Here's the drawing with two shaded views (mm, measured from the low corner). I have some questions. A direction names the side the tool comes from. Round coordinates to 2 decimals unless told otherwise and drop trailing zeros. Write each loop counter-clockwise with the first axis right and the second up, starting at its lowest first coordinate (ties: lowest second). Pieces come first, ordered by that corner, then holes. Notation, with made-up numbers: M -31,5.25 L 25,5.25 A24 ccw 25,40.25 Z; hole C 37.5,-5 d11. An arc over 180 degrees is marked long. Write item = value, one per line. Start each with the question number.
(1) I want a section at B-B (z = 7.5). List the corners of the cut face in (x, y) for me.
(2) I want a section at D-D (y = 3). List the corners of the cut face in (x, z) for me.
(3) Will these pins go through, and if not, where does the flat tip stop? pin 1 Ø6 at (x, z) = (17, 5) entering from +Y; pin 2 Ø0.7 at (x, y) = (18.5, 0) entering from +Z; pin 3 Ø1.5 at (y, z) = (8, 4) entering from +X; pin 4 Ø3.5 at (x, z) = (17.5, 8.5) entering from -Y.
(4) I want a section at C-C (x = 17). List the corners of the cut face in (y, z) for me.
(5) I want a section at A-A (x = 30.75). List the corners of the cut face in (y, z) for me.
(6) On a 3-axis mill with a long thin cutter (end or side, diameter ignored), from which of +Z, -Z, +X, -X, +Y, -Y can I reach the whole of each face in a straight line? I mean the marked faces 1, 2 and 3. Say none if no direction works.
(7) If we mould it in two halves opening along X, with no side actions, what happens to the marked faces 4, 5 and 6? For each: released by +X, released by -X, zero draft, split by the parting line, or undercut.
(8) I need wall thicknesses on line 1 along X through (y, z) = (9.5, 5); line 2 along Y through (x, z) = (32.5, 2.75); line 3 along X through (y, z) = (8.5, 8.5). Which ranges of each line are inside material? Lowest first, please.
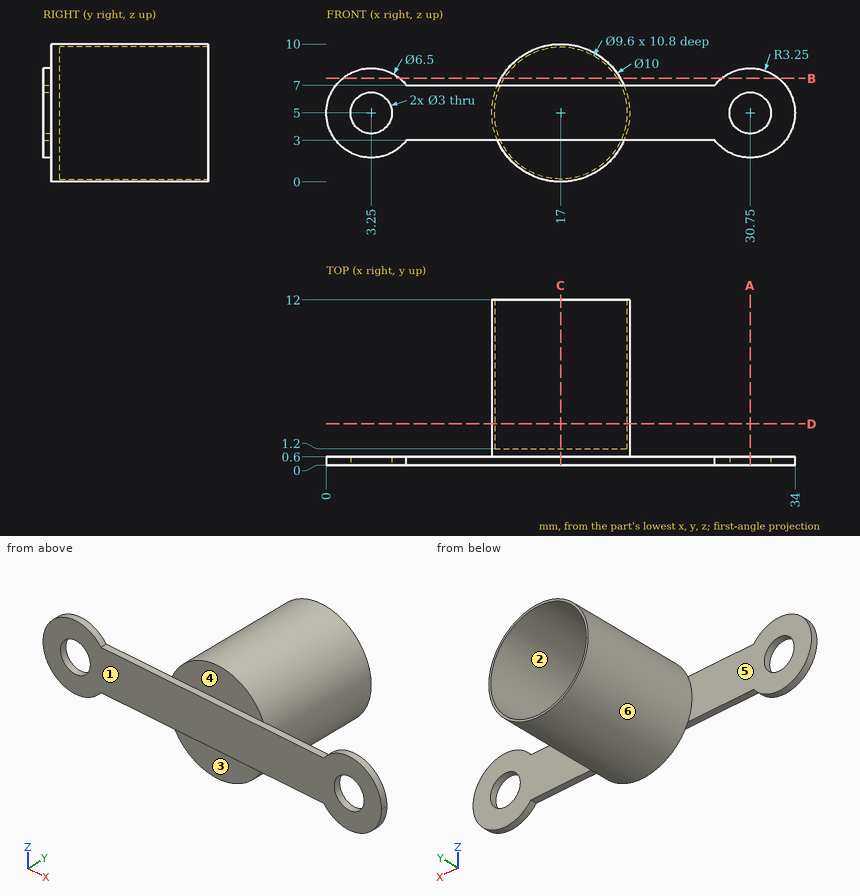
Returned:
q1.outline = M 1.17,0 L 5.33,0 L 5.33,0.6 L 1.17,0.6 Z; M 12.67,0.6 L 21.33,0.6 L 21.33,12 L 21.1,12 L 21.1,1.2 L 12.9,1.2 L 12.9,12 L 12.67,12 Z; M 28.67,0 L 32.83,0 L 32.83,0.6 L 28.67,0.6 Z
q2.outline = C 17,5 d10; hole C 17,5 d9.6
q3.pin_1 = 1.2
q3.pin_2 = 7
q3.pin_3 = 21.99
q3.pin_4 = 0
q4.outline = M 0,3 L 0.6,3 L 0.6,0 L 12,0 L 12,0.2 L 1.2,0.2 L 1.2,9.8 L 12,9.8 L 12,10 L 0.6,10 L 0.6,7 L 0,7 Z
q5.outline = M 0,1.75 L 0.6,1.75 L 0.6,3.5 L 0,3.5 Z; M 0,6.5 L 0.6,6.5 L 0.6,8.25 L 0,8.25 Z
q6.face_1 = +Z, -Z, +X, -X, -Y
q6.face_2 = +Y
q6.face_3 = -Z, -Y
q7.face_4 = undercut
q7.face_5 = zero draft
q7.face_6 = split by the parting line
q8.line_1 = 12 to 12.2, 21.8 to 22
q8.line_2 = 0 to 0.6
q8.line_3 = 13.43 to 13.72, 20.28 to 20.57
